```python
from build123d import *

# Parameters (mm, degrees)
BOSS_EXTRUDE1_DEPTH    = 18
CUT_EXTRUDE1_DEPTH     = 23
F_12_0MM_DOWEL_HOLE3_D = 9
CUT_EXTRUDE5_DEPTH     = 36


with BuildPart() as part:
    # Sketch1 → Boss-Extrude1 (new body, symmetric)
    with BuildSketch(Plane.XY):
        with BuildLine():
            Line((18.027756377, 6), (22, 6))
            Line((22, 6), (22, 19))
            Line((22, 19), (50, 19))
            Line((50, 19), (50, 28))
            Line((50, 28), (25.690465157, 28))
            ThreePointArc((25.690465157, 28), (0, 38), (-25.690465157, 28))
            Line((-25.690465157, 28), (-50, 28))
            Line((-50, 28), (-50, 19))
            Line((-50, 19), (-22, 19))
            Line((-22, 19), (-22, 6))
            Line((-22, 6), (-18.027756377, 6))
            ThreePointArc((-18.027756377, 6), (0, 19), (18.027756377, 6))
        make_face()
    extrude(amount=BOSS_EXTRUDE1_DEPTH, both=True)

    # Sketch3 → Cut-Extrude1 (cut, through all)
    with BuildSketch(Plane(origin=(0, 28, 0), x_dir=(1, 0, 0), z_dir=(0, 1, 0))):
        with BuildLine():
            Line((-44.497190923, 18), (-50, 18))
            Line((-50, 18), (-50, -18))
            Line((-50, -18), (-44.497190923, -18))
            ThreePointArc((-44.497190923, -18), (-48, 0), (-44.497190923, 18))
        make_face()
    cut_extrude1 = extrude(amount=-CUT_EXTRUDE1_DEPTH, mode=Mode.SUBTRACT)

    # Ø12.0mm Dowel Hole3 (through all)
    with Locations(Plane(origin=(0, 28, 0), x_dir=(1, 0, 0), z_dir=(0, 1, 0))):
        with Locations((-31, 0)):
            f_12_0mm_dowel_hole3 = Hole(F_12_0MM_DOWEL_HOLE3_D / 2)

    # Sketch17 → Cut-Extrude5 (cut)
    with BuildSketch(Plane(origin=(0, 28, 0), x_dir=(1, 0, 0), z_dir=(0, 1, 0))):
        with BuildLine():
            Line((-25.690465157, -6.637683312), (-25.690465157, 6.637683312))
            ThreePointArc((-25.690465157, 6.637683312), (-22.5, 0), (-25.690465157, -6.637683312))
        make_face()
    cut_extrude5 = extrude(amount=CUT_EXTRUDE5_DEPTH, mode=Mode.SUBTRACT)

    # Sketch20 → CBORE for M6 Hex Head Bolt1 (revolve, cut)
    with BuildSketch(Plane(origin=(0, 38, -2.983943356), x_dir=(0, 0, 1), z_dir=(1, 0, 0))):
        Polygon((0, 0), (0, 32), (2.5, 32), (2.5, 13.495), (2.995, 13), (3, 13), (3, 0), align=None)
    cbore_for_m6_hex_head_bolt1 = revolve(axis=Axis((0, 44.35, -2.983943356), (0, -1, 0)), mode=Mode.SUBTRACT)

    # Mirror1: Cut-Extrude1, Ø12.0mm Dowel Hole3, Cut-Extrude5, CBORE for M6 Hex Head Bolt1 across plane
    add(cut_extrude1.mirror(Plane(origin=(0, 0, 0), x_dir=(0, 0, 1), z_dir=(1, 0, 0))), mode=Mode.SUBTRACT)
    add(f_12_0mm_dowel_hole3.mirror(Plane(origin=(0, 0, 0), x_dir=(0, 0, 1), z_dir=(1, 0, 0))), mode=Mode.SUBTRACT)
    add(cut_extrude5.mirror(Plane(origin=(0, 0, 0), x_dir=(0, 0, 1), z_dir=(1, 0, 0))), mode=Mode.SUBTRACT)
    add(cbore_for_m6_hex_head_bolt1.mirror(Plane(origin=(0, 0, 0), x_dir=(0, 0, 1), z_dir=(1, 0, 0))), mode=Mode.SUBTRACT)


solid = part.part
```
Check sheet for the modelled part. Datum: model origin and axes. Units: mm. A direction names the side the tool comes from. Round coordinates to 2 decimals unless told otherwise and drop trailing zeros. Order: outer loops, then holes, each group sorted by start corner. A loop starts at its lowest first (then second) coordinate and runs counter-clockwise, first axis right, second up. Notation, with made-up numbers: (31.5, 58.25) - (56.5, 58.25) arc R31 ccw to (56.5, 90.25) - close; hole circle Ø9 at (19, -12.5). An arc over 180 degrees is marked (long way). Write item = value, one per line.
Q1. Section check A-A (y = 21.5). Record the boundary of the cut face in (x, z).
Computed:
outline = (-44.5, -18) - (44.5, -18) arc R48 ccw to (44.5, 18) - (-44.5, 18) arc R48 ccw to start; hole circle Ø9 at (-31, 0); hole circle Ø5 at (0, -2.98); hole circle Ø9 at (31, 0)
Q2. Section check D-D (x = 0). Record the boundary of the cut face in (y, z) (3 decimals), and give its area (3 significant figures).
Computed:
outline = (19, -18) - (38, -18) - (38, -5.984) - (25, -5.984) - (25, -5.979) - (24.505, -5.484) - (19, -5.484) - close; (19, -0.484) - (24.505, -0.484) - (25, 0.011) - (25, 0.016) - (38, 0.016) - (38, 18) - (19, 18) - close
area = 576 mm^2
Q3. Draft check along X on faces 1 (the face through (1.149, 31.591, -0.213)), 2 (the face through (0.395, 37.998, 0.252)), 3 (the face through (1.52, 21.71, -4.97)), 4 (the face through (-20, 6, 0)). Enter one of: pulls with the +X half, pulls with the -X half, needs draft (parallel to the pull), parting line crosses it, or undercut.
Computed:
face_1 = undercut
face_2 = parting line crosses it
face_3 = undercut
face_4 = needs draft
Q4. Go/stop test with flat-tipped pins: pin 1 (6 mm diameter, centred on x = -33, z = 3, fed in from +Y); pin 2 (6 mm diameter, centred on x = 0, z = -2.98, fed in from -Y); pin 3 (4 mm diameter, centred on y = 15.5, z = -5.5, fed in from -X). Record where each tip stops, or that it passes through.
Computed:
pin_1 = 28
pin_2 = 18.76
pin_3 = -22
Q5. Tool access check on faces 5 (the face through (38, 19, 0)), 6 (the face through (22.5, 29, -0.1)), 7 (the face through (-22.5, 29, -0.1)), 8 (the face through (-38, 19, 0)). Record the directions out of +Z, -Z, +X, -X, +Y, -Y that give a thin tool (end or side, any length) a straight path to the whole face; none if there is none.
Computed:
face_5 = +Z, -Z, +X, -Y
face_6 = +X, +Y
face_7 = -X, +Y
face_8 = +Z, -Z, -X, -Y
Q6. Section check C-C (y = 13.5). Record the boundary of the cut face in (x, z).
Computed:
outline = (-22, -18) - (-13.37, -18) - (-13.37, 18) - (-22, 18) - close; (13.37, -18) - (22, -18) - (22, 18) - (13.37, 18) - close
Q7. Thickness scan on line 1 along Z through (x, y) = (-31, 24); line 2 along Z through (x, y) = (0, 22.1); line 3 along Y through (x, z) = (40, -8). Record the ranges inside material, lowest first.
Computed:
line_1 = -18 to -4.5, 4.5 to 18
line_2 = -18 to -5.48, -0.48 to 18
line_3 = 19 to 28
Q8. Section check B-B (x = -31). Record the boundary of the cut face in (y, z).
Computed:
outline = (19, -18) - (28, -18) - (28, -4.5) - (19, -4.5) - close; (19, 4.5) - (28, 4.5) - (28, 18) - (19, 18) - close
